Autodesk Inventor part; units mm, degrees
ref_plane "YZ Plane" through (0, 0, 0) normal (1, 0, 0) x (0, 1, 0)
ref_plane "XZ Plane" through (0, 0, 0) normal (0, 1, 0) x (-1, 0, 0)
ref_plane "XY Plane" through (0, 0, 0) normal (0, 0, 1) x (1, 0, 0)
sketch "Sketch1" plane through (0, 0, 0) normal (0, 1, 0) x (-1, 0, 0)
  circle A0 centre (0, 0) radius 2.1
  line L0 (0, -3.9007) -> (-2.84, -3.9007)
  line L1 (-5.4993, -8.2) -> (-3.1, -8.2)
  line L2 (-3.1, -8.2) -> (-4.9, -10)
  line L3 (-4.9, -10) -> (-10, -10)
  line L4 (-10, -10) -> (-10, -4.9)
  line L5 (-10, -4.9) -> (-8.2, -3.1)
  line L6 (-8.2, -3.1) -> (-8.2, -5.4993)
  line L7 (-3.9007, -2.84) -> (-3.9007, 0)
  line L8 (-3.9007, 0) -> (-2.1, 0)
  line L9 (0, -3.9007) -> (0, -2.1) construction
  line L10 (-5.4993, -8.2) -> (-5.4993, -6.56)
  line L11 (-5.4993, -6.56) -> (-2.84, -3.9007)
  line L12 (-3.9007, -2.84) -> (-6.56, -5.4993)
  line L13 (-6.56, -5.4993) -> (-8.2, -5.4993)
  line L14 (6.56, -5.4993) -> (3.9007, -2.84)
  line L15 (3.1, -8.2) -> (5.4993, -8.2)
  line L16 (5.4993, -6.56) -> (5.4993, -8.2)
  line L17 (8.2, -5.4993) -> (8.2, -3.1)
  line L18 (8.2, -5.4993) -> (6.56, -5.4993)
  line L19 (8.2, -3.1) -> (10, -4.9)
  line L20 (4.9, -10) -> (3.1, -8.2)
  line L21 (10, -4.9) -> (10, -10)
  line L22 (10, -10) -> (4.9, -10)
  line L23 (2.84, -3.9007) -> (0, -3.9007)
  line L24 (0, -3.9007) -> (0, -2.1) construction
  line L25 (3.9007, 0) -> (2.1, 0)
  line L26 (3.9007, 0) -> (3.9007, -2.84)
  line L27 (2.84, -3.9007) -> (5.4993, -6.56)
  line L28 (5.4993, 6.56) -> (2.84, 3.9007)
  line L29 (8.2, 3.1) -> (8.2, 5.4993)
  line L30 (6.56, 5.4993) -> (8.2, 5.4993)
  line L31 (5.4993, 8.2) -> (3.1, 8.2)
  line L32 (5.4993, 8.2) -> (5.4993, 6.56)
  line L33 (3.1, 8.2) -> (4.9, 10)
  line L34 (10, 4.9) -> (8.2, 3.1)
  line L35 (4.9, 10) -> (10, 10)
  line L36 (10, 10) -> (10, 4.9)
  line L37 (3.9007, 2.84) -> (3.9007, 0)
  line L38 (3.9007, 0) -> (2.1, 0) construction
  line L39 (0, 3.9007) -> (0, 2.1)
  line L40 (0, 3.9007) -> (2.84, 3.9007)
  line L41 (3.9007, 2.84) -> (6.56, 5.4993)
  line L42 (-6.56, 5.4993) -> (-3.9007, 2.84)
  line L43 (-3.1, 8.2) -> (-5.4993, 8.2)
  line L44 (-5.4993, 6.56) -> (-5.4993, 8.2)
  line L45 (-8.2, 5.4993) -> (-8.2, 3.1)
  line L46 (-8.2, 5.4993) -> (-6.56, 5.4993)
  line L47 (-8.2, 3.1) -> (-10, 4.9)
  line L48 (-4.9, 10) -> (-3.1, 8.2)
  line L49 (-10, 4.9) -> (-10, 10)
  line L50 (-10, 10) -> (-4.9, 10)
  line L51 (-2.84, 3.9007) -> (0, 3.9007)
  line L52 (0, 3.9007) -> (0, 2.1) construction
  line L53 (-3.9007, 0) -> (-2.1, 0) construction
  line L54 (-3.9007, 0) -> (-3.9007, 2.84)
  line L55 (-2.84, 3.9007) -> (-5.4993, 6.56)
  point P0 (0, -3.0003)
  point P1 (-3.0003, 0)
  point P2 (0, -3.0003)
  point P3 (3.0003, 0)
  point P4 (3.0003, 0)
  point P5 (0, 3.0003)
  point P6 (0, 3.0003)
  point P7 (-3.0003, 0)
  dimension "d0" = 4.2
  dimension "d2" = 45
  dimension "d3" = 3.1
  dimension "d4" = 2.84
  dimension "d7" = 10
  dimension "d8" = 10
  dimension "d9" = 1.5
  dimension "d10" = 1.8
  dimension "d11" = 1.64
  dimension "d14" = 360
extrude "Extrusion1" add sketch "Sketch1" along normal mid plane 25 contours L25 L26 L14 L18 L17 L19 L21 L22 L20 L15 L16 L27 L23 L0 L11 L10 L1 L2 L3 L4 L5 L6 L13 L12 L7 L8 A0 | A0 L39 L40 L28 L32 L31 L33 L35 L36 L34 L29 L30 L41 L37 L25 | A0 L8 L54 L42 L46 L45 L47 L49 L50 L48 L43 L44 L55 L51 L39
properties part number "vslot_25mm" material "Aluminum 6061-AHC"
Part model, mm, in its own coordinate system. A direction names the side the tool comes from. Give positions to 0.01 mm unless a question says otherwise; leave off trailing zeros. Order: outer loops, then holes, each group sorted by start corner. A loop starts at its lowest first (then second) coordinate and runs counter-clockwise, first axis right, second up. Notation, with made-up numbers: M 70,44.5 L 122,44.5 A32 ccw 122,75.5 Z; hole C 34.25,49.5 d7. An arc over 180 degrees is marked long. Use a Markdown table: item, result. Add a question column.
(1) Saw through at A-A, the plane x = 0. Give the cut face in (y, z), and give its area (3 significant figures).
(2) 3-axis set-ups, long thin cutter, end or side, ignore diameter. For faces 4 (the face through (0, 0, -3.901)), 5 (the face through (8.2, 0, 4)), 6 (the face through (9.1, -0.2, -4)), 7 (the face through (-3.901, 0, 0)): which of +Z, -Z, +X, -X, +Y, -Y reach the whole face in a straight line?
(3) Drop flat-ended pins along their axis: P1, Ø2, axis at y = -9.5, z = -2.5, coming from the +X side; P2, Ø1.2, axis at y = 0, z = -4, coming from the -X side; P3, Ø3, axis at x = 0, y = -5, coming from the -Z side. Give the stop position or say it passes through.
(4) Probe line 1 along Z through (x, y) = (-9, -3); line 2 along X through (y, z) = (-4.75, 0). List the from-to ranges inside material, lowest first. Write a range as [from, to].
(5) Mould opens along X. For faces 1 (the face through (0.1, 12.5, 2.4)), 2 (the face through (-4, -0.2, 9.1)), 3 (the face through (-10, 0, 7)) say: +X half, -X half, draft (parallel to the pull), parting line (faces both ways), or undercut.
(6) Saw through at B-B, the plane z = 0. Give the cut face in (x, y).
Answer key:
| question | item | result |
|---|---|---|
| 1 | outline | M -12.5,-3.9 L 12.5,-3.9 L 12.5,-2.1 L -12.5,-2.1 Z; M -12.5,2.1 L 12.5,2.1 L 12.5,3.9 L -12.5,3.9 Z |
| 1 | area | 90.0 mm^2 |
| 2 | face 4 | -Z, +Y, -Y |
| 2 | face 5 | +Y, -Y |
| 2 | face 6 | +X, +Y, -Y |
| 2 | face 7 | -X, +Y, -Y |
| 3 | P1 | x = 8.6 |
| 3 | P2 | x = -9.7 |
| 3 | P3 | z = -3.9 |
| 4 | line 1 | [-10, -3.9], [3.9, 10] |
| 4 | line 2 | [-3.9, -2.1], [2.1, 3.9] |
| 5 | face 1 | draft |
| 5 | face 2 | undercut |
| 5 | face 3 | -X half |
| 6 | outline | M -3.9,-12.5 L -2.1,-12.5 L -2.1,12.5 L -3.9,12.5 Z; M 2.1,-12.5 L 3.9,-12.5 L 3.9,12.5 L 2.1,12.5 Z |
